from build123d import *

# Parameters (mm, degrees)
SKETCH1_W           = 50.8
SKETCH1_H           = 457.2
BOSS_EXTRUDE1_DEPTH = 50.8
SHELL1_T            = -2.54
SKETCH2_W           = 45.72
SKETCH2_H           = 45.72
CUT_EXTRUDE1_DEPTH  = 50.8


with BuildPart() as part:
    # Sketch1 → Boss-Extrude1 (new body)
    with BuildSketch(Plane.XY):
        with Locations((25.4, -228.6)):
            Rectangle(SKETCH1_W, SKETCH1_H)
    extrude(amount=BOSS_EXTRUDE1_DEPTH)

    # Shell1
    shell1_openings = [part.faces().sort_by_distance(p)[0] for p in [
        (25.4, 0, 25.4),
    ]]
    offset(amount=SHELL1_T, openings=shell1_openings, kind=Kind.INTERSECTION)

    # Sketch2 → Cut-Extrude1 (cut)
    with BuildSketch(Plane.XZ.offset(457.2)):
        with Locations((25.4, 25.4)):
            Rectangle(SKETCH2_W, SKETCH2_H)
    extrude(amount=-CUT_EXTRUDE1_DEPTH, mode=Mode.SUBTRACT)


solid = part.part
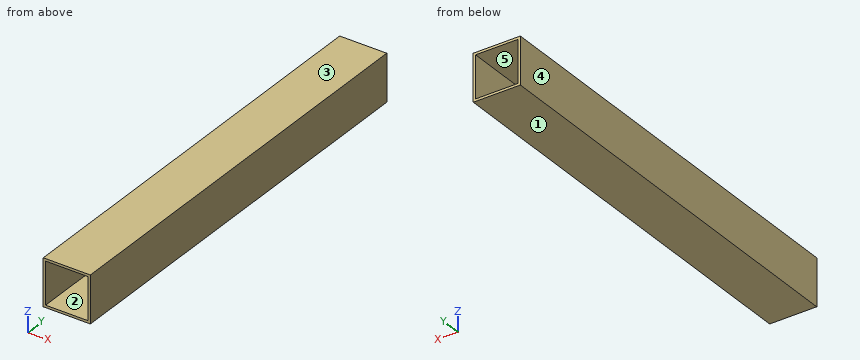
Build history of the part. All positions in model axes, mm. Face numbers are marked on the shaded views. A direction names the side the tool comes from. Give positions to 0.01 mm unless a question says otherwise; leave off trailing zeros. Loops run counter-clockwise (first coordinate to the right, second up) from the corner with the lowest first, then second, coordinate; pieces in that order, holes last. Notation, with made-up numbers: (-40, -29.75) -> (-34, -29.75) arc R30 cw to (-34, 2.25) -> close; hole circle Ø1 at (82.25, 30.25). An arc over 180 degrees is marked (long way). Answer in a Markdown table with one row per item.
Item 1: Slice it at B-B on x = 18.5. Write the cut outline in (y, z).
Findings below:
| item | result |
|---|---|
| outline | (-457.2, 0) -> (0, 0) -> (0, 2.54) -> (-457.2, 2.54) -> close; (-457.2, 48.26) -> (0, 48.26) -> (0, 50.8) -> (-457.2, 50.8) -> close |
Item 2: Flat gauge pin, fed straight in: P1, Ø13.5, axis at y = -142, z = 23, coming from the -X side. Where does the tip first touch, or does it go through?
Findings below:
| item | result |
|---|---|
| P1 | stops at x = 0 |
Item 3: Slice it at C-C on z = 17.5. Write the cut outline in (x, y), plus the area to 3 significant figures.
Findings below:
| item | result |
|---|---|
| outline | (0, -457.2) -> (2.54, -457.2) -> (2.54, 0) -> (0, 0) -> close; (48.26, -457.2) -> (50.8, -457.2) -> (50.8, 0) -> (48.26, 0) -> close |
| area | 2,320 mm² |
Item 4: Probe line 1 along X through (y, z) = (-188.5, 33.5). List the from-to ranges inside material, lowest first. Write a range as [from, to].
Findings below:
| item | result |
|---|---|
| line 1 | x = [0, 2.54], [48.26, 50.8] |
Item 5: Mould opens along X. For the marked faces 3, 4 and 5 say: pulls with the +X half, pulls with the -X half, needs draft (parallel to the pull), parting line crosses it, or undercut.
Findings below:
| item | result |
|---|---|
| face 3 | needs draft |
| face 4 | pulls with the -X half |
| face 5 | undercut |
Item 6: Tool access for the marked faces 1 and 2: list every direction of +Z, -Z, +X, -X, +Y, -Y with a clear straight run to the whole face (end or side of a thin tool).
Findings below:
| item | result |
|---|---|
| face 1 | -Z, +X, -X, +Y, -Y |
| face 2 | +Y, -Y |
Item 7: Slice it at A-A on y = -121.5. Write the cut outline in (x, z), plus the area to 3 significant figures.
Findings below:
| item | result |
|---|---|
| outline | (0, 0) -> (50.8, 0) -> (50.8, 50.8) -> (0, 50.8) -> close; hole (2.54, 2.54) -> (48.26, 2.54) -> (48.26, 48.26) -> (2.54, 48.26) -> close |
| area | 490 mm² |
